Geometry check sheet. Reference: the model listing, model coordinates, mm. Face numbers are marked on the shaded views. A direction names the side the tool comes from. Coordinates: 2 decimals unless noted, no trailing zeros. Write each loop counter-clockwise with the first axis right and the second up, starting at its lowest first coordinate (ties: lowest second). Pieces come first, ordered by that corner, then holes. Notation, with made-up numbers: M -9.75,32.25 L 43.25,32.25 A11 cw 43.25,38.25 Z; hole C 49,79 d2. An arc over 180 degrees is marked long. Put each result on its own line as item: value. Start each with the question number.
1) Scan lines: line 1 along Z through (x, y) = (-20, -15.5); line 2 along Z through (x, y) = (-13.5, -26.5); line 3 along X through (y, z) = (-12, -75). Record each from-to range of solid material in increasing order.
2) Mould release check, pull along X, two halves, no side actions. Record for the marked faces 3, 4, 5 and 6: released by +X, released by -X, zero draft, split by the parting line, or undercut.
3) Cross-section at B-B on z = -59. Record the cut outline in (x, y).
4) Cross-section at A-A on x = 12.16. Record the cut outline in (y, z).
5) Set-up check for the marked faces 1 and 2: record each of +Z, -Z, +X, -X, +Y, -Y from which the full face is reachable in a straight line by a thin tool's end or side.
6) Gauge pin test, flat ends, axial feed: pin 1 (1.5 mm diameter, centred on x = 17, z = -72, fed in from +Y); pin 2 (1.5 mm diameter, centred on x = 11, z = -34.5, fed in from +Y). Record the tip position at first contact, or that the pin passes through.
7) Cross-section at D-D on x = -20. Record the cut outline in (y, z).
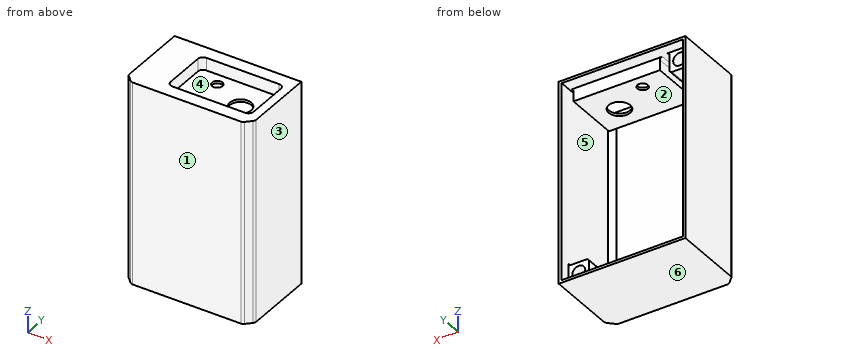
from build123d import *

# Parameters (mm, degrees)
F1_W      = 50
F1_H      = 27.68
F1_W_2    = 47.8036555797
F1_H_2    = 25.68
F2_DEPTH  = 80
F1_W_3    = 34.129309468
F1_H_3    = 21.4303236678
F1_W_4    = 32.75
F1_H_4    = 20.5
F3_DEPTH  = 6
F0_W      = 32.75
F0_H      = 20.5
F0_R      = 2.05
F0_R_2    = 4.25
F4_DEPTH  = 6
F5_DEPTH  = 5
F6_DEPTH  = 1
F7_R      = 2
F8_W      = 50
F8_H      = 80
F9_DEPTH  = 1
F10_ANGLE = 180
F11_W     = 47.8036555797
F11_H     = 25.68
F12_DEPTH = 1
F13_W     = 8
F13_H     = 8
F14_DEPTH = 8
F15_W     = 8
F15_H     = 8
F16_DEPTH = 8
F19_SIZE  = 2
F20_SIZE  = 3
F21_R     = 1.5
F22_R     = 1
F18_R     = 2.55
F23_DEPTH = 5.1
F24_W     = 50
F24_H     = 80
F25_DEPTH = 4.18


with BuildPart() as f2:
    # F1 (on face) → F2 (new body)
    with BuildSketch(Plane.XY):
        Rectangle(F1_W, F1_H)
        with Locations((-0.0981722102, 0)):
            Rectangle(F1_W_2, F1_H_2, mode=Mode.SUBTRACT)
    extrude(amount=F2_DEPTH)

    # F8 (on face) → F9 (cut)
    with BuildSketch(Plane.XZ.offset(13.84)):
        with Locations((0, 40)):
            Rectangle(F8_W, F8_H)
    extrude(amount=-F9_DEPTH, mode=Mode.SUBTRACT)


with BuildPart() as f3:
    # F1 (on face) → F3 (new body)
    with BuildSketch(Plane.XY):
        with Locations((5.3276410885, -1.4191564249)):
            Rectangle(F1_W_3, F1_H_3)
        with Locations((5.28, -1.59)):
            Rectangle(F1_W_4, F1_H_4, mode=Mode.SUBTRACT)
    extrude(amount=F3_DEPTH)

    # F0 (on Top) → F4 (join)
    with BuildSketch(Plane.XY):
        with Locations((5.28, -1.59)):
            Rectangle(F0_W, F0_H)
        with Locations((-1.515, -6.89)):
            Circle(F0_R, mode=Mode.SUBTRACT)
        with Locations((12.16, 0)):
            Circle(F0_R_2, mode=Mode.SUBTRACT)
    extrude(amount=F4_DEPTH)

    # F1 (on face) → F5 (cut)
    with BuildSketch(Plane.XY):
        with Locations((5.28, -1.59)):
            Rectangle(F1_W_4, F1_H_4)
    extrude(amount=F5_DEPTH, mode=Mode.SUBTRACT)

    # F7
    f7_edges = [f3.edges().sort_by_distance(p)[0] for p in [
        (21.655, -11.84, 2.5),
        (-11.095, -11.84, 2.5),
        (21.655, 8.66, 2.5),
        (-11.095, 8.66, 2.5),
    ]]
    fillet(f7_edges, radius=F7_R)


with BuildPart() as f6:
    # F1 (on face) → F6 (new body)
    with BuildSketch(Plane.XY):
        with Locations((-0.0981722102, 0)):
            Rectangle(F1_W_2, F1_H_2)
        with Locations((5.3276410885, -1.4191564249)):
            Rectangle(F1_W_3, F1_H_3, mode=Mode.SUBTRACT)
    extrude(amount=F6_DEPTH)


with BuildPart() as f6_1:
    # F10: moved
    add(f6.part.rotate(Axis((-0.0981722102, -12.84, 0), (1, 0, 0)), F10_ANGLE))


with BuildPart() as f2_1:
    # F10: moved
    add(f2.part.rotate(Axis((-0.0981722102, -12.84, 0), (1, 0, 0)), F10_ANGLE))

    # F11 (on face) → F12 (join)
    with BuildSketch(Plane(origin=(0, 0, -80), x_dir=(1, 0, 0), z_dir=(0, 0, -1))):
        with Locations((-0.0981722102, 25.68)):
            Rectangle(F11_W, F11_H)
    extrude(amount=-F12_DEPTH)


    add(f6_1.part)  # F14 merges F6
    # F13 (on face) → F14 (join)
    with BuildSketch(Plane.YZ.offset(-24)):
        with Locations((-16.84, -5)):
            Rectangle(F13_W, F13_H)
    extrude(amount=F14_DEPTH)

    # F15 (on face) → F16 (join)
    with BuildSketch(Plane(origin=(23.8036555797, 0, 0), x_dir=(0, -1, 0), z_dir=(-1, 0, 0))):
        with Locations((16.84, -75)):
            Rectangle(F15_W, F15_H)
    extrude(amount=F16_DEPTH)


with BuildPart() as f3_1:
    # F10: moved
    add(f3.part.rotate(Axis((-0.0981722102, -12.84, 0), (1, 0, 0)), F10_ANGLE))


with BuildPart() as f2_2:
    add(f2_1.part)

    # F17: union F3
    add(f3_1.part)

    # F19
    f19_edges = [f2_2.edges().sort_by_distance(p)[0] for p in [
        (23.803656, -38.52, -40),
        (-24, -38.52, -40),
    ]]
    chamfer(f19_edges, length=F19_SIZE)

    # F20
    f20_edges = [f2_2.edges().sort_by_distance(p)[0] for p in [
        (-25, -39.52, -40),
        (25, -39.52, -40),
    ]]
    chamfer(f20_edges, length=F20_SIZE)

    # F21
    f21_edges = [f2_2.edges().sort_by_distance(p)[0] for p in [
        (25, -36.52, -40),
        (22, -39.52, -40),
        (-22, -39.52, -40),
        (-25, -36.52, -40),
    ]]
    fillet(f21_edges, radius=F21_R)

    # F22
    f22_edges = [f2_2.edges().sort_by_distance(p)[0] for p in [
        (-24, -16.84, -9),
        (-20, -20.84, -9),
        (-16, -16.84, -9),
        (-16, -20.84, -5),
        (-16, -16.84, -1),
        (15.803656, -16.84, -71),
        (23.803656, -16.84, -71),
        (15.803656, -16.84, -79),
        (15.803656, -20.84, -75),
        (19.803656, -20.84, -71),
        (-11.737014, -24.260844, -1),
        (22.392296, -24.260844, -1),
        (-20, -20.84, -1),
        (23.803656, -20.84, -75),
        (19.803656, -20.84, -79),
        (-24, -20.84, -5),
    ]]
    fillet(f22_edges, radius=F22_R)

    # F18 (on face) → F23 (cut)
    with BuildSketch(Plane(origin=(0, -12.84, 0), x_dir=(-1, 0, 0), z_dir=(0, 1, 0))):
        with Locations((20, -5)):
            Circle(F18_R)
        with Locations((-19.8036555797, -75)):
            Circle(F18_R)
    extrude(amount=-F23_DEPTH, mode=Mode.SUBTRACT)

    # F24 (on face) → F25 (join)
    with BuildSketch(Plane(origin=(0, -12.84, 0), x_dir=(-1, 0, 0), z_dir=(0, 1, 0))):
        with Locations((0, -40)):
            Rectangle(F24_W, F24_H)
        Polygon((-23.8036555797, -70), (-23.8036555797, -1), (15, -1), (24, -1), (24, -10), (24, -79), (-14.8036555797, -79), (-23.8036555797, -79), align=None, mode=Mode.SUBTRACT)
    extrude(amount=F25_DEPTH)


solid = f2_2.part
Answer key:
1. line 1: z = -80 to -79, -9 to -7.55, -2.45 to 0
1. line 2: z = -80 to -79, -1 to 0
1. line 3: x = -25 to -24, 23.8 to 25
2. face 3: released by +X
2. face 4: undercut
2. face 5: undercut
2. face 6: zero draft
3. outline: M -25,-35.9 A1.5 ccw -24.56,-36.96 L -22.44,-39.08 A1.5 ccw -21.38,-39.52 L 21.38,-39.52 A1.5 ccw 22.44,-39.08 L 24.56,-36.96 A1.5 ccw 25,-35.9 L 25,-8.66 L 23.8,-8.66 L 23.8,-36.52 L 21.8,-38.52 L -22,-38.52 L -24,-36.52 L -24,-8.66 L -25,-8.66 Z
4. outline: M -39.52,-80 L -8.66,-80 L -8.66,-79 L -38.52,-79 L -38.52,-1 L -34.98,-1 L -34.98,-6 L -29.93,-6 L -29.93,-5 L -34.34,-5 L -34.34,0 L -39.52,0 Z; M -21.43,-6 L -13.55,-6 L -13.55,-1 L -8.66,-1 L -8.66,0 L -13.84,0 L -13.84,-5 L -21.43,-5 Z
5. face 1: +Z, -Z, +X, -X, -Y
5. face 2: +Y
6. pin 1: stops at y = -12.84
6. pin 2: stops at y = -38.52
7. outline: M -39.52,-80 L -8.66,-80 L -8.66,-79 L -38.52,-79 L -38.52,-1 L -21.84,-1 A1 cw -20.84,-2 L -20.84,-8 A1 ccw -19.84,-9 L -12.84,-9 L -12.84,-7.55 L -17.94,-7.55 L -17.94,-2.45 L -12.84,-2.45 L -12.84,-1 L -8.66,-1 L -8.66,0 L -39.52,0 Z
